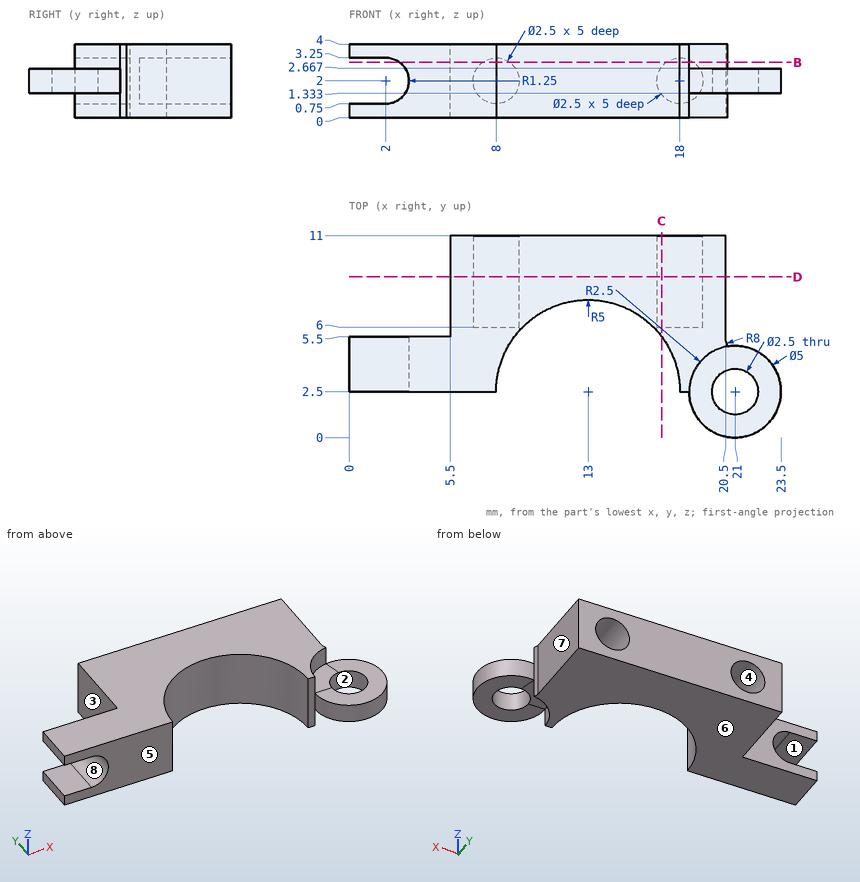
Could you check a few things on this drawing? It's one solid part, dimensions in mm from its lowest x, y, z. A direction names the side the tool comes from. Coordinates: 2 decimals unless noted, no trailing zeros. Loops run counter-clockwise (first coordinate to the right, second up) from the corner with the lowest first, then second, coordinate; pieces in that order, holes last.
1. For the marked faces 1, 2, 3, 4 and 5, which set-ups out of +Z, -Z, +X, -X, +Y, -Y let a thin tool reach every point of the face, with its end or its side?
2. We'd pull the mould along Z, two halves only. Please class the marked faces 6, 7 and 8: released by +Z, released by -Z, zero draft, split by the parting line, or undercut.
3. Imagine slicing it at D-D (y = 8.75). Please give me the cut outline in (x, z).
4. Imagine slicing it at C-C (x = 17). Please give me the cut outline in (y, z), and give its area (3 significant figures).
5. I need wall thicknesses on L1, parallel to X at y = 9, z = 2.1; L2, parallel to X at y = 7, z = 2.3 (1 decimal); L3, parallel to Z at x = 18, y = 9.5. Which ranges of each line are inside material? Lowest first, please.
6. Imagine slicing it at B-B (z = 3). Please give me the cut outline in (x, y).
7. For P1, Ø1.5, axis at x = 21, y = 1, coming from the +Z side; P2, Ø1, axis at y = 3, z = 1, coming from the +X side; P3, Ø5.5, axis at x = 21.5, y = 2, coming from the -Z side, each with a flat end and sliding along its axis, tell me the tip position at first contact or that it passes through.
Computed values:
1. face 1: -X, +Y, -Y
1. face 2: +Z, -Z
1. face 3: +Z, -Z, -X, +Y
1. face 4: +Y
1. face 5: +Z, -Z, -X, -Y
2. face 6: released by -Z
2. face 7: zero draft
2. face 8: undercut
3. outline: (5.5, 0) - (20.5, 0) - (20.5, 4) - (5.5, 4) - close; hole circle Ø2.5 at (8, 2); hole circle Ø2.5 at (18, 2)
4. outline: (5.5, 0) - (11, 0) - (11, 1.25) - (6, 1.25) - (6, 2.75) - (11, 2.75) - (11, 4) - (5.5, 4) - close
4. area: 14.5 mm2
5. L1: x = 5.5 to 6.75, 9.25 to 16.75, 19.25 to 20.5
5. L2: x = 5.5 to 6.8, 9.2 to 10.8, 15.2 to 16.8, 19.2 to 20.5
5. L3: z = 0 to 0.75, 3.25 to 4
6. outline: (2.75, 2.5) - (8, 2.5) arc R5 cw to (18, 2.5) - (18.5, 2.5) arc R2.5 cw to (20.61, 4.97) arc R8 ccw to (20.5, 5.28) - (20.5, 11) - (18.75, 11) - (18.75, 6) - (17.25, 6) - (17.25, 11) - (8.75, 11) - (8.75, 6) - (7.25, 6) - (7.25, 11) - (5.5, 11) - (5.5, 5.5) - (2.75, 5.5) - close
7. P1: stops at z = 2.67
7. P2: stops at x = 23.5
7. P3: stops at z = 1.33
